Model file for the job. Use its own axes, mm. Face numbers are marked on the shaded views. A direction names the side the tool comes from. Round coordinates to 2 decimals unless told otherwise and drop trailing zeros. Loops run counter-clockwise (first coordinate to the right, second up) from the corner with the lowest first, then second, coordinate; pieces in that order, holes last. Notation, with made-up numbers: M 20,-20.75 L 41,-20.75 A22 cw 41,-5.75 Z; hole C 18.5,45 d9. An arc over 180 degrees is marked long. Use a Markdown table: item, result. Add a question column.
Item 1: Tool access for the marked faces 1 and 2: list every direction of +Z, -Z, +X, -X, +Y, -Y with a clear straight run to the whole face (end or side of a thin tool).
Item 2: Saw through at B-B on z = 2.75. Write the cut outline in (x, y).
Item 3: Pin check, flat tips, straight feed: P1, Ø4.5, axis at x = 0, y = -4.17, coming from the +Z side; P2, Ø1.5, axis at x = -5, y = 6.5, coming from the +Z side; P3, Ø3, axis at x = 6, y = 6, coming from the +Z side. Stop position of each tip, or through.
Item 4: Saw through at D-D on x = 8.5. Write the cut outline in (y, z), then the cut area to 3 significant figures.
Item 5: Saw through at C-C on y = -5.25. Write the cut outline in (x, z).
Item 6: Saw through at A-A on x = 0. Write the cut outline in (y, z).
Item 7: Two-plate mould, pull along Y, no slides. Class the marked faces 3, 4 and 5: +Y half, -Y half, draft (parallel to the pull), parting line (faces both ways), or undercut.
Item 8: Wall check: L1, parallel to Y at x = 0, z = 5; L2, parallel to Z at x = -3.5, y = 2; L3, parallel to X at y = -4.5, z = 3.75. Give the ranges that are in metal, low to high. Write a range as from..to.
```python
from build123d import *

# Parameters (mm, degrees)
SKETCH_1_W          = 24.1
SKETCH_1_H          = 20
EXTRUDE_1_DEPTH     = 13
CUT_EXTRUDE_2_DEPTH = 30.151500819
SKETCH_4_R          = 2
CUT_EXTRUDE_3_DEPTH = 21.351965507
CUT_EXTRUDE_4_DEPTH = 27.724567349
SKETCH_6_R          = 2
CUT_EXTRUDE_5_DEPTH = 30.151500819


with BuildPart() as part:
    # 草图1 → 凸台-拉伸1 (new body)
    with BuildSketch(Plane.XY):
        Rectangle(SKETCH_1_W, SKETCH_1_H)
    extrude(amount=EXTRUDE_1_DEPTH)

    # 草图3 → 切除-拉伸2 (cut, through all)
    with BuildSketch(Plane(origin=(12.05, 0, 0), x_dir=(0, 0, -1), z_dir=(1, 0, 0))):
        with BuildLine():
            Line((-0.7940006, 10), (-13, 10))
            Line((-13, 10), (-13, 1.657184567))
            ThreePointArc((-13, 1.657184567), (-6.535745695, 5.300056859), (-0.7940006, 10))
        make_face()
    extrude(amount=-CUT_EXTRUDE_2_DEPTH, mode=Mode.SUBTRACT)

    # 草图4 → 切除-拉伸3 (cut, through all)
    with BuildSketch(Plane.XY.offset(13)):
        with Locations((0, -4.171407716)):
            Circle(SKETCH_4_R)
    extrude(amount=-CUT_EXTRUDE_3_DEPTH, mode=Mode.SUBTRACT)

    # 草图5 → 切除-拉伸4 (cut, through all)
    with BuildSketch(Plane.XZ.offset(10)):
        Polygon((0, 13), (-8.05, 13), (-4, 7), (0, 7), align=None)
        Polygon((8.05, 13), (0, 13), (0, 7), (4, 7), align=None)
    extrude(amount=-CUT_EXTRUDE_4_DEPTH, mode=Mode.SUBTRACT)

    # 草图6 → 切除-拉伸5 (cut, through all)
    with BuildSketch(Plane(origin=(12.05, 0, 0), x_dir=(0, 0, -1), z_dir=(1, 0, 0))):
        with Locations(Location((-4, 2, 0), (0, 0, 90))):
            Circle(SKETCH_6_R)
    extrude(amount=-CUT_EXTRUDE_5_DEPTH, mode=Mode.SUBTRACT)


solid = part.part
```
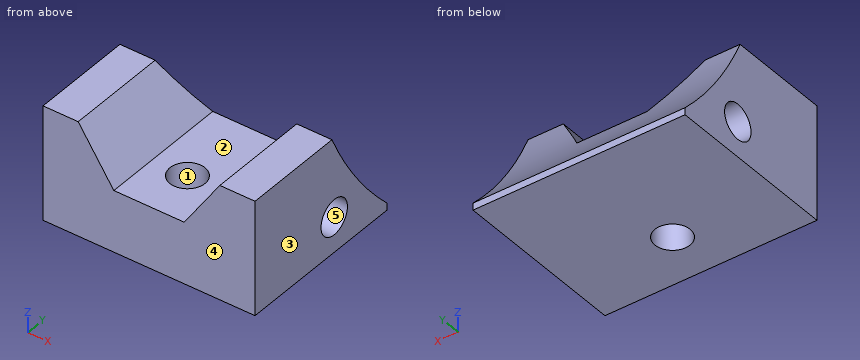
Entries:
| question | item | result |
|---|---|---|
| 1 | face 1 | +Z, -Z |
| 1 | face 2 | +Z, +Y, -Y |
| 2 | outline | M -12.05,-10 L 12.05,-10 L 12.05,0.44 L -12.05,0.44 Z; M -12.05,3.56 L 12.05,3.56 L 12.05,8.21 L -12.05,8.21 Z; hole C 0,-4.17 d4 |
| 3 | P1 | z = 7 |
| 3 | P2 | z = 5.89 |
| 3 | P3 | z = 7.75 |
| 4 | outline | M -10,0 L 10,0 L 10,0.79 A43 cw 1.66,13 L -10,13 Z; hole C 2,4 d4 |
| 4 | area | 190 mm2 |
| 5 | outline | M -12.05,0 L -1.68,0 L -1.68,7 L -4,7 L -8.05,13 L -12.05,13 Z; M 1.68,0 L 12.05,0 L 12.05,13 L 8.05,13 L 4,7 L 1.68,7 Z |
| 6 | outline | M -10,0 L -6.17,0 L -6.17,7 L -10,7 Z; M -2.17,0 L 10,0 L 10,0.79 A43 cw 4.99,7 L -2.17,7 Z; hole C 2,4 d4 |
| 7 | face 3 | draft |
| 7 | face 4 | -Y half |
| 7 | face 5 | undercut |
| 8 | L1 | -10..-6.17, -2.17..0.27, 3.73..6.4 |
| 8 | L2 | 0..2, 6..7 |
| 8 | L3 | -12.05..-1.97, 1.97..12.05 |
